Source: CAD feature listing. Evaluate the final solid. Frame: model axes, mm. Face numbers are marked on the shaded views. A direction names the side the tool comes from. Round coordinates to 2 decimals unless told otherwise and drop trailing zeros. Write each loop counter-clockwise with the first axis right and the second up, starting at its lowest first coordinate (ties: lowest second). Pieces come first, ordered by that corner, then holes. Notation, with made-up numbers: M -29.5,-21 L -5.5,-21 A27 cw -5.5,15 Z; hole C 43.25,-32 d9. An arc over 180 degrees is marked long. Answer in a Markdown table with one row per item.
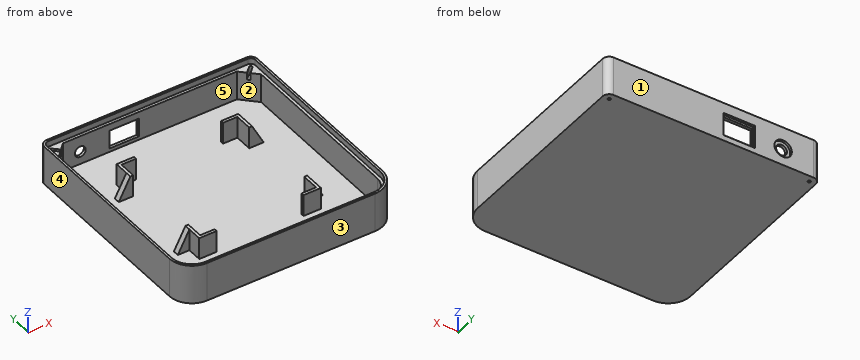
from build123d import *

# Parameters (mm, degrees)
BOSS_EXTRUDE1_DEPTH = 3
BOSS_EXTRUDE2_DEPTH = 20
CHAMFER1_SIZE       = 10
SKETCH3_W           = 84
SKETCH3_H           = 84
SKETCH3_W_2         = 80
SKETCH3_H_2         = 80
BOSS_EXTRUDE3_DEPTH = 15
BOSS_EXTRUDE4_DEPTH = 84
SKETCH7_W           = 8
SKETCH7_H           = 10
SKETCH7_H_2         = 56
SKETCH7_W_2         = 60
SKETCH7_H_3         = 84
CUT_EXTRUDE1_DEPTH  = 72
FILLET1_R           = 3
BOSS_EXTRUDE5_DEPTH = 27
SKETCH10_R          = 3.75
CUT_EXTRUDE2_DEPTH  = 26
CUT_EXTRUDE3_DEPTH  = 5
SKETCH12_R          = 1
CUT_EXTRUDE4_DEPTH  = 33
SKETCH14_R          = 6
CUT_EXTRUDE5_DEPTH  = 1.6
SKETCH15_W          = 20.5
SKETCH15_H          = 12.8
CUT_EXTRUDE6_DEPTH  = 9.6
SKETCH16_W          = 22
SKETCH16_H          = 16
CUT_EXTRUDE7_DEPTH  = 1.6
SKETCH18_W          = 84
SKETCH18_H          = 56
CUT_EXTRUDE8_DEPTH  = 15


with BuildPart() as part:
    # Sketch1 → Boss-Extrude1 (new body)
    with BuildSketch(Plane.XY):
        with BuildLine():
            Line((58, -72), (-58, -72))
            ThreePointArc((-58, -72), (-67.899494937, -67.899494937), (-72, -58))
            Line((-72, -58), (-72, 72))
            Line((-72, 72), (72, 72))
            Line((72, 72), (72, -58))
            ThreePointArc((72, -58), (67.899494937, -67.899494937), (58, -72))
        make_face()
    extrude(amount=BOSS_EXTRUDE1_DEPTH)

    # Sketch2 → Boss-Extrude2 (add)
    with BuildSketch(Plane.XY.offset(3)):
        with BuildLine():
            Line((-72, 72), (-72, -58))
            ThreePointArc((-72, -58), (-67.899494937, -67.899494937), (-58, -72))
            Line((-58, -72), (58, -72))
            ThreePointArc((58, -72), (67.899494937, -67.899494937), (72, -58))
            Line((72, -58), (72, 72))
            Line((72, 72), (-72, 72))
        make_face()
        with BuildLine():
            Line((-70, 70), (-70, -58))
            ThreePointArc((-70, -58), (-66.485281374, -66.485281374), (-58, -70))
            Line((-58, -70), (58, -70))
            ThreePointArc((58, -70), (66.485281374, -66.485281374), (70, -58))
            Line((70, -58), (70, 70))
            Line((70, 70), (-70, 70))
        make_face(mode=Mode.SUBTRACT)
    extrude(amount=BOSS_EXTRUDE2_DEPTH)

    # Chamfer1
    chamfer1_edges = [part.edges().sort_by_distance(p)[0] for p in [
        (-70, 70, 13),
        (70, 70, 13),
    ]]
    chamfer(chamfer1_edges, length=CHAMFER1_SIZE)

    # Sketch3 → Boss-Extrude3 (add)
    with BuildSketch(Plane.XY.offset(3)):
        Rectangle(SKETCH3_W, SKETCH3_H)
        Rectangle(SKETCH3_W_2, SKETCH3_H_2, mode=Mode.SUBTRACT)
    extrude(amount=BOSS_EXTRUDE3_DEPTH)

    # Sketch6 → Boss-Extrude4 (add)
    with BuildSketch(Plane.XZ.offset(42)):
        Polygon((-42, 3), (-50, 3), (-42, 18), align=None)
        Polygon((42, 18), (42, 3), (50, 3), align=None)
    extrude(amount=-BOSS_EXTRUDE4_DEPTH)

    # Sketch7 → Cut-Extrude1 (cut)
    with BuildSketch(Plane.XY.offset(3)):
        with Locations((-46, 37)):
            Rectangle(SKETCH7_W, SKETCH7_H)
        with Locations((-46, 0)):
            Rectangle(SKETCH7_W, SKETCH7_H_2)
        with Locations((-46, -37)):
            Rectangle(SKETCH7_W, SKETCH7_H)
        with Locations((46, -37)):
            Rectangle(SKETCH7_W, SKETCH7_H)
        with Locations((46, 0)):
            Rectangle(SKETCH7_W, SKETCH7_H_2)
        with Locations((46, 37)):
            Rectangle(SKETCH7_W, SKETCH7_H)
        Rectangle(SKETCH7_W_2, SKETCH7_H_3)
    extrude(amount=CUT_EXTRUDE1_DEPTH, mode=Mode.SUBTRACT)

    # Fillet1
    fillet1_edges = [part.edges().sort_by_distance(p)[0] for p in [
        (-72, 72, 11.5),
        (72, 72, 11.5),
    ]]
    fillet(fillet1_edges, radius=FILLET1_R)

    # Sketch9 → Boss-Extrude5 (add)
    with BuildSketch(Plane(origin=(0, 0, 0), x_dir=(-1, 0, 0), z_dir=(0, 0, -1))):
        with BuildLine():
            Line((73.5, -58), (73.5, 69))
            ThreePointArc((73.5, 69), (72.181980515, 72.181980515), (69, 73.5))
            Line((69, 73.5), (-69, 73.5))
            ThreePointArc((-69, 73.5), (-72.181980515, 72.181980515), (-73.5, 69))
            Line((-73.5, 69), (-73.5, -58))
            ThreePointArc((-73.5, -58), (-68.960155108, -68.960155108), (-58, -73.5))
            Line((-58, -73.5), (58, -73.5))
            ThreePointArc((58, -73.5), (68.960155108, -68.960155108), (73.5, -58))
        make_face()
        with BuildLine():
            Line((72, -58), (72, 69))
            ThreePointArc((72, 69), (71.121320344, 71.121320344), (69, 72))
            Line((69, 72), (-69, 72))
            ThreePointArc((-69, 72), (-71.121320344, 71.121320344), (-72, 69))
            Line((-72, 69), (-72, -58))
            ThreePointArc((-72, -58), (-67.899494937, -67.899494937), (-58, -72))
            Line((-58, -72), (58, -72))
            ThreePointArc((58, -72), (67.899494937, -67.899494937), (72, -58))
        make_face(mode=Mode.SUBTRACT)
    extrude(amount=-BOSS_EXTRUDE5_DEPTH)

    # Sketch10 → Cut-Extrude2 (cut)
    with BuildSketch(Plane.XZ.offset(-70)):
        with Locations((-48, 11.832723103)):
            Circle(SKETCH10_R)
    extrude(amount=-CUT_EXTRUDE2_DEPTH, mode=Mode.SUBTRACT)

    # Sketch11 → Cut-Extrude3 (cut)
    with BuildSketch(Plane.XY.offset(23)):
        with BuildLine():
            Line((-69.688606392, 68.274864677), (-65.603988879, 64.396011121))
            Line((-65.603988879, 64.396011121), (-64.178908017, 65.821091983))
            Line((-64.178908017, 65.821091983), (-68.242386769, 69.652703755))
            ThreePointArc((-68.242386769, 69.652703755), (-69.689783022, 69.724016148), (-69.688606392, 68.274864677))
        make_face()
        with BuildLine():
            Line((64.178908017, 65.821091983), (65.603988879, 64.396011121))
            Line((65.603988879, 64.396011121), (69.688606392, 68.274864677))
            ThreePointArc((69.688606392, 68.274864677), (69.689783022, 69.724016148), (68.242386769, 69.652703755))
            Line((68.242386769, 69.652703755), (64.178908017, 65.821091983))
        make_face()
    extrude(amount=-CUT_EXTRUDE3_DEPTH, mode=Mode.SUBTRACT)

    # Sketch12 → Cut-Extrude4 (cut)
    with BuildSketch(Plane.XY.offset(18)):
        with Locations((-69, 69)):
            Circle(SKETCH12_R)
        with Locations((69, 69)):
            Circle(SKETCH12_R)
    extrude(amount=-CUT_EXTRUDE4_DEPTH, mode=Mode.SUBTRACT)

    # Sketch14 → Cut-Extrude5 (cut)
    with BuildSketch(Plane(origin=(0, 73.5, 0), x_dir=(1, 0, 0), z_dir=(0, 1, 0))):
        with Locations(Location((-48, -11.832723103, 0), (0, 0, 270))):
            Circle(SKETCH14_R)
    extrude(amount=-CUT_EXTRUDE5_DEPTH, mode=Mode.SUBTRACT)

    # Sketch15 → Cut-Extrude6 (cut)
    with BuildSketch(Plane(origin=(0, 73.5, 0), x_dir=(1, 0, 0), z_dir=(0, 1, 0))):
        with Locations((-17.75, -11.832723103)):
            Rectangle(SKETCH15_W, SKETCH15_H)
    extrude(amount=-CUT_EXTRUDE6_DEPTH, mode=Mode.SUBTRACT)

    # Sketch16 → Cut-Extrude7 (cut)
    with BuildSketch(Plane(origin=(0, 73.5, 0), x_dir=(1, 0, 0), z_dir=(0, 1, 0))):
        with Locations((-17.75, -11.832723103)):
            Rectangle(SKETCH16_W, SKETCH16_H)
    extrude(amount=-CUT_EXTRUDE7_DEPTH, mode=Mode.SUBTRACT)

    # Sketch18 → Cut-Extrude8 (cut)
    with BuildSketch(Plane.XY.offset(18)):
        Rectangle(SKETCH18_W, SKETCH18_H)
    extrude(amount=-CUT_EXTRUDE8_DEPTH, mode=Mode.SUBTRACT)


solid = part.part
Q1. Material intervals for probe 1 along Y at (x, z) = (56.5, 5); probe 2 along Y at (x, z) = (-27, 5.25), sorted ascending.
Solutions:
| item | result |
|---|---|
| probe 1 | y = -73.5 to -70, 70 to 73.5 |
| probe 2 | y = -73.5 to -70, 70 to 71.9 |
Q2. Pull-direction query (X, two-part tool) for the marked faces 3, 4 and 5; classes: pulls with the +X half, pulls with the -X half, needs draft (parallel to the pull), parting line crosses it, or undercut.
Solutions:
| item | result |
|---|---|
| face 3 | needs draft |
| face 4 | pulls with the -X half |
| face 5 | undercut |
Q3. Contact query for flat-ended pins moving along their axis: pin 1 Ø1.3 at (y, z) = (72.5, 16) entering from -X; pin 2 Ø12 at (x, y) = (20.5, 23.5) entering from +Z; pin 3 Ø2 at (y, z) = (71.5, 15) entering from -X. Output: stop coordinate, or through.
Solutions:
| item | result |
|---|---|
| pin 1 | stops at x = -72.48 |
| pin 2 | stops at z = 3 |
| pin 3 | stops at x = -73.24 |
Q4. Access query for the marked faces 1 and 2. Directions: +Z, -Z, +X, -X, +Y, -Y. A direction counts if a zero-diameter tool reaches every point of the face in a straight line with its end or side. Return the directions, or none.
Solutions:
| item | result |
|---|---|
| face 1 | +Z, -Z, +X, -X, +Y |
| face 2 | +Z |
Q5. Section A-A (x = -14). Return loops of the section in (y, z), and give its area (3 significant figures).
Solutions:
| item | result |
|---|---|
| outline | M -73.5,0 L 73.5,0 L 73.5,3.83 L 71.9,3.83 L 71.9,5.43 L 70,5.43 L 70,3 L -70,3 L -70,23 L -72,23 L -72,27 L -73.5,27 Z; M 70,18.23 L 71.9,18.23 L 71.9,19.83 L 73.5,19.83 L 73.5,27 L 72,27 L 72,23 L 70,23 Z |
| area | 543 mm2 |
Q6. Section C-C (x = -35.5). Return loops of the section in (y, z), and give its area (3 significant figures).
Solutions:
| item | result |
|---|---|
| outline | M -73.5,0 L 73.5,0 L 73.5,27 L 72,27 L 72,23 L 70,23 L 70,3 L 42,3 L 42,18 L 40,18 L 40,3 L -40,3 L -40,18 L -42,18 L -42,3 L -70,3 L -70,23 L -72,23 L -72,27 L -73.5,27 Z |
| area | 653 mm2 |
Q7. Section B-B (y = -4). Return loops of the section in (x, z).
Solutions:
| item | result |
|---|---|
| outline | M -73.5,0 L 73.5,0 L 73.5,27 L 72,27 L 72,23 L 70,23 L 70,3 L -70,3 L -70,23 L -72,23 L -72,27 L -73.5,27 Z |
